```python
from build123d import *

# Parameters (mm, degrees)
SKETCH1_R           = 27.5
BOSS_EXTRUDE1_DEPTH = 9.525
BOSS_EXTRUDE2_START = -3.175
SKETCH2_R           = 20
SKETCH2_R_2         = 2
BOSS_EXTRUDE2_DEPTH = 3.175
SKETCH8_R           = 2
CUT_EXTRUDE6_DEPTH  = 52.5


with BuildPart() as part:
    # Sketch1 → Boss-Extrude1 (new body)
    with BuildSketch(Plane.XY):
        with BuildLine():
            Line((-30.675000233, 40), (-30.675000233, -40))
            ThreePointArc((-30.675000233, -40), (0, -70.675000233), (30.675000233, -40))
            Line((30.675000233, -40), (30.675000233, 40))
            ThreePointArc((30.675000233, 40), (0, 70.675000233), (-30.675000233, 40))
        make_face()
        with Locations(Location((0, 40, 0), (0, 0, 180))):
            Circle(SKETCH1_R, mode=Mode.SUBTRACT)
        with Locations(Location((0, -40, 0), (0, 0, 180))):
            Circle(SKETCH1_R, mode=Mode.SUBTRACT)
    extrude(amount=BOSS_EXTRUDE1_DEPTH)

    # Sketch2 → Boss-Extrude2 (add)
    with BuildSketch(Plane.XY.offset(9.525).offset(BOSS_EXTRUDE2_START)):
        with BuildLine():
            Line((-30.675000233, 40), (-30.675000233, -40))
            ThreePointArc((-30.675000233, -40), (0, -70.675000233), (30.675000233, -40))
            Line((30.675000233, -40), (30.675000233, 40))
            ThreePointArc((30.675000233, 40), (0, 70.675000233), (-30.675000233, 40))
        make_face()
        with Locations((0, 40)):
            Circle(SKETCH2_R, mode=Mode.SUBTRACT)
        with Locations((0, 64)):
            Circle(SKETCH2_R_2, mode=Mode.SUBTRACT)
        with Locations((20.784609691, 52)):
            Circle(SKETCH2_R_2, mode=Mode.SUBTRACT)
        with Locations((20.784609691, 28)):
            Circle(SKETCH2_R_2, mode=Mode.SUBTRACT)
        with Locations((0, 16)):
            Circle(SKETCH2_R_2, mode=Mode.SUBTRACT)
        with Locations((-20.784609691, 28)):
            Circle(SKETCH2_R_2, mode=Mode.SUBTRACT)
        with Locations((-20.784609691, 52)):
            Circle(SKETCH2_R_2, mode=Mode.SUBTRACT)
        with Locations(Location((-20.784609691, -52, 0), (0, 0, 180))):
            Circle(SKETCH2_R_2, mode=Mode.SUBTRACT)
        with Locations(Location((-20.784609691, -28, 0), (0, 0, 180))):
            Circle(SKETCH2_R_2, mode=Mode.SUBTRACT)
        with Locations(Location((0, -16, 0), (0, 0, 180))):
            Circle(SKETCH2_R_2, mode=Mode.SUBTRACT)
        with Locations(Location((20.784609691, -28, 0), (0, 0, 180))):
            Circle(SKETCH2_R_2, mode=Mode.SUBTRACT)
        with Locations(Location((20.784609691, -52, 0), (0, 0, 180))):
            Circle(SKETCH2_R_2, mode=Mode.SUBTRACT)
        with Locations(Location((0, -64, 0), (0, 0, 180))):
            Circle(SKETCH2_R_2, mode=Mode.SUBTRACT)
        with Locations(Location((0, -40, 0), (0, 0, 180))):
            Circle(SKETCH2_R, mode=Mode.SUBTRACT)
    extrude(amount=BOSS_EXTRUDE2_DEPTH)

    # Sketch8 → Cut-Extrude6 (cut, symmetric)
    with BuildSketch(Plane(origin=(0, 0, 0), x_dir=(0, 0, -1), z_dir=(1, 0, 0))):
        with Locations((-4.7625, 0)):
            Circle(SKETCH8_R)
    extrude(amount=CUT_EXTRUDE6_DEPTH, both=True, mode=Mode.SUBTRACT)


solid = part.part
```
Input: part model. Units: mm. Frame: model coordinates. A direction names the side the tool comes from. Coordinates: 2 decimals unless noted, no trailing zeros. Write each loop counter-clockwise with the first axis right and the second up, starting at its lowest first coordinate (ties: lowest second). Pieces come first, ordered by that corner, then holes. Notation, with made-up numbers: (45, 86.5) - (62, 86.5) arc R23 cw to (62, 114.5) - close; hole circle Ø6 at (9, 15). An arc over 180 degrees is marked (long way). Put each result on its own line as item: value. Start each with the question number.
1) Cut plane D-D (y = -52). Return the cut outline in (x, z) (3 decimals), plus the area to 3 significant figures.
2) Cut plane C-C (x = 15.5). State how many separate pieces and enclosed holes the cut face has, plus the area to 3 significant figures.
3) Cut plane B-B (y = 0). Return the cut outline in (x, z) (1 decimal), plus the area to 3 significant figures.
4) Cut plane A-A (z = 4). Return the cut outline in (x, y) (3 decimals), plus the area to 3 significant figures.
5) Contact query for flat-ended pins moving along their axis: pin 1 (2.5 mm diameter, centred on x = 0, y = -64, fed in from +Z); pin 2 (5 mm diameter, centred on x = 20.78, y = 28, fed in from -Z); pin 3 (1.5 mm diameter, centred on x = 4.5, z = 1.5, fed in from -Y); pin 4 (5 mm diameter, centred on x = 0.5, z = 2, fed in from +Y) (3 decimals). Output: stop coordinate, or through.
6) Mould query, pull axis X, two halves, no side actions, for faces 1 (the face through (-30.675, 1, 7)), 2 (the face through (0, 1, 9.525)), 3 (the face through (21.22, -26.05, 7.92)). Classes: pulls with the +X half, pulls with the -X half, needs draft (parallel to the pull), parting line crosses it, or undercut.
7) Reachability of faces 4 (the face through (-26.23, -48.26, 3.13)), 5 (the face through (0.429, -1.774, 3.84)) from +Z, -Z, +X, -X, +Y, -Y: full face, straight path, thin tool, end or side. Return the list, or none.
8) Ray query, L1, parallel to Y at x = -15.5, z = 8.5; L2, parallel to Y at x = 0, z = 4.25 (3 decimals); L3, parallel to Y at x = -12, z = 5.25. Return the intervals inside material, ascending.
Resolved:
1. outline: (-28.23, 0) - (-24.744, 0) - (-24.744, 6.35) - (-22.785, 6.35) - (-22.785, 9.525) - (-28.23, 9.525) - close; (-18.785, 6.35) - (-16, 6.35) - (-16, 9.525) - (-18.785, 9.525) - close; (16, 6.35) - (18.785, 6.35) - (18.785, 9.525) - (16, 9.525) - close; (22.785, 6.35) - (24.744, 6.35) - (24.744, 0) - (28.23, 0) - (28.23, 9.525) - (22.785, 9.525) - close
1. area: 96.5 mm2
2. separate pieces: 3
2. enclosed holes: 1
2. area: 516 mm2
3. outline: (-30.7, 0) - (30.7, 0) - (30.7, 2.8) - (-30.7, 2.8) - close; (-30.7, 6.8) - (30.7, 6.8) - (30.7, 9.5) - (-30.7, 9.5) - close
3. area: 339 mm2
4. outline: (-30.675, -40) arc R30.675 ccw to (30.675, -40) - (30.675, -1.849) - (-30.675, -1.849) - close; (-30.675, 1.849) - (30.675, 1.849) - (30.675, 40) arc R30.675 ccw to (-30.675, 40) - close; hole circle Ø55 at (0, -40); hole circle Ø55 at (0, 40)
4. area: 2,890 mm2
5. pin 1: passes through
5. pin 2: stops at z = 6.35
5. pin 3: stops at y = -70.44
5. pin 4: stops at y = 70.675
6. face 1: pulls with the -X half
6. face 2: needs draft
6. face 3: undercut
7. face 4: -Z
7. face 5: +X, -X
8. L1: y = -66.47 to -52.64, -27.36 to 27.36, 52.64 to 66.47
8. L2: y = -70.675 to -67.5, -12.5 to -1.933, 1.933 to 12.5, 67.5 to 70.675
8. L3: y = -68.23 to -64.74, -15.26 to -1.94, 1.94 to 15.26, 64.74 to 68.23
